Verification items for the finished model (mm, model axes). A direction names the side the tool comes from. Round coordinates to 2 decimals unless told otherwise and drop trailing zeros. Write each loop counter-clockwise with the first axis right and the second up, starting at its lowest first coordinate (ties: lowest second). Pieces come first, ordered by that corner, then holes. Notation, with made-up numbers: M 85,71 L 114,71 A29 ccw 114,97 Z; hole C 13,58 d6. An arc over 180 degrees is marked long. One line per item, written item: value. Start each with the question number.
Item 1: Section check B-B, the plane y = -67. Record the cut outline in (x, z), then the cut area to 3 significant figures.
Item 2: Thickness scan on probe 1 along Y at (x, z) = (13.5, -36); probe 2 along X at (y, z) = (-36, -20); probe 3 along Z at (x, y) = (26.5, -51.5). Record the ranges inside material, lowest first. Write a range as from..to.
Item 3: Gauge pin test, flat end, axial feed: pin 1 (8 mm diameter, centred on x = 18, y = -60.5, fed in from +Z). Record the tip position at first contact, or that the pin passes through.
Item 4: Section check C-C, the plane x = 21.5. Record the cut outline in (y, z).
Item 5: Tool access check on faces 1 (the face through (-10, -12.7, 1)), 2 (the face through (-13, -95, 48.157)). Record the directions out of +Z, -Z, +X, -X, +Y, -Y that give a thin tool (end or side, any length) a straight path to the whole face; none if there is none.
Item 6: Draft check along Y on faces 3 (the face through (-8.68, -1.45, 46.63)), 4 (the face through (-10, -50, -54.188)), 5 (the face through (30.67, -51.4, 46.71)), 6 (the face through (-10, -101.6, -2)). Enter one of: +Y half, -Y half, draft (parallel to the pull), parting line (faces both ways), or undercut.
Item 7: Section check A-A, the plane z = 18. Record the cut outline in (x, y).
from build123d import *

# Parameters (mm, degrees)
F0_W         = 102.3449450731
F0_H         = 102.3449450731
F1_DEPTH     = 101.6
F2_T         = -12.7
F3_R         = 5.08
F4_T1_DEPTH  = 92.1849450731
F4_T3_DEPTH  = 92.1849450731
F4_T5_DEPTH  = 91.44
F4_S9_W      = 5.08
F4_S9_H      = 5.08
F4_T10_DEPTH = 5.08
F4_S15_W     = 5.08
F4_S15_H     = 5.08
F4_T16_DEPTH = 5.08
F4_S21_W     = 5.08
F4_S21_H     = 5.08
F4_T22_DEPTH = 5.08
F4_S27_W     = 5.08
F4_S27_H     = 5.08
F4_T28_DEPTH = 5.08
F4_T32_ANGLE = 90
F4_T34_ANGLE = 90


# Not quite as in the source:
# - a fillet or chamfer that OpenCascade refuses, or shapes differently, is made with other operations: its cross-section is extruded or revolved along the edge and cut away or added


with BuildPart() as f1:
    # F0 (on Front) → F1 (new body)
    with BuildSketch(Plane.XZ):
        with Locations((-9.3297921121, -3.0156895518)):
            Rectangle(F0_W, F0_H)
    extrude(amount=F1_DEPTH)

    # F2
    f2_openings = [f1.faces().sort_by_distance(p)[0] for p in [
        (-9.329792, -50.8, 48.156783),
    ]]
    offset(amount=F2_T, openings=f2_openings)

    # F3
    f3_edges = [f1.edges().sort_by_distance(p)[0] for p in [
        (41.84268, -50.8, 48.156783),
        (-9.329792, -101.6, 48.156783),
        (41.84268, -101.6, -3.01569),
        (41.84268, -50.8, -54.188162),
        (-9.329792, -101.6, -54.188162),
        (-9.329792, -88.9, 48.156783),
        (-60.502265, -50.8, 48.156783),
        (-9.329792, 0, 48.156783),
        (29.14268, -50.8, 48.156783),
        (-9.329792, -12.7, 48.156783),
        (-47.802265, -50.8, 48.156783),
    ]]
    fillet(f3_edges, radius=F3_R)

    # F4: fillet of radius 5.08 on 3 edges, made by hand

    # F4_s2 → F4_t1 (cut)
    with BuildSketch(Plane.YZ.offset(-55.4222646487)):
        with BuildLine():
            ThreePointArc((-5.08, -54.1881620884), (-1.4878975516, -52.7002645368), (0, -49.1081620884))
            Line((0, -49.1081620884), (0, -54.1881620884))
            Line((0, -54.1881620884), (-5.08, -54.1881620884))
        make_face()
    extrude(amount=F4_T1_DEPTH, mode=Mode.SUBTRACT)

    # F4_s4 → F4_t3 (cut)
    with BuildSketch(Plane.XY.offset(-49.1081620884)):
        with BuildLine():
            ThreePointArc((-60.5022646487, -5.08), (-59.0143670971, -1.4878975516), (-55.4222646487, 0))
            Line((-55.4222646487, 0), (-60.5022646487, 0))
            Line((-60.5022646487, 0), (-60.5022646487, -5.08))
        make_face()
        with BuildLine():
            ThreePointArc((-60.5022646487, -96.52), (-59.0143670971, -100.1121024484), (-55.4222646487, -101.6))
            Line((-55.4222646487, -101.6), (-60.5022646487, -101.6))
            Line((-60.5022646487, -101.6), (-60.5022646487, -96.52))
        make_face()
        with BuildLine():
            ThreePointArc((36.7626804245, 0), (40.3547828729, -1.4878975516), (41.8426804245, -5.08))
            Line((41.8426804245, -5.08), (41.8426804245, 0))
            Line((41.8426804245, 0), (36.7626804245, 0))
        make_face()
    extrude(amount=F4_T3_DEPTH, mode=Mode.SUBTRACT)

    # F4_s6 → F4_t5 (cut)
    with BuildSketch(Plane.XZ.offset(5.08)):
        with BuildLine():
            ThreePointArc((-60.5022646487, -49.1081620884), (-59.0143670971, -52.7002645368), (-55.4222646487, -54.1881620884))
            Line((-55.4222646487, -54.1881620884), (-60.5022646487, -54.1881620884))
            Line((-60.5022646487, -54.1881620884), (-60.5022646487, -49.1081620884))
        make_face()
    extrude(amount=F4_T5_DEPTH, mode=Mode.SUBTRACT)


with BuildPart() as f4_tool8:
    # F4_s9 → F4_t10 (new body)
    with BuildSketch(Plane.YZ.offset(-55.4222646487)):
        with Locations((-99.06, 45.6167829847)):
            Rectangle(F4_S9_W, F4_S9_H)
    extrude(amount=-F4_T10_DEPTH)

    # F4_s11 → F4_t12 (revolve, cut)
    with BuildSketch(Plane(origin=(-55.4222646487, -96.52, 43.0767829847), x_dir=(0, 0.7071067812, -0.7071067812), z_dir=(0, 0.7071067812, 0.7071067812))):
        with BuildLine():
            ThreePointArc((0, -5.08), (5.08, 0), (0, 5.08))
            Line((0, 5.08), (0, -5.08))
        make_face()
    revolve(axis=Axis((-55.4222646487, -96.52, 43.0767829847), (-1, 0, 0)), mode=Mode.SUBTRACT)


with BuildPart() as f1_1:
    add(f1.part)

    # F4_t7: cut F4_tool8
    add(f4_tool8.part, mode=Mode.SUBTRACT)


with BuildPart() as f4_tool14:
    # F4_s15 → F4_t16 (new body)
    with BuildSketch(Plane.YZ.offset(-55.4222646487)):
        with Locations((-2.54, 45.6167829847)):
            Rectangle(F4_S15_W, F4_S15_H)
    extrude(amount=-F4_T16_DEPTH)

    # F4_s17 → F4_t18 (revolve, cut)
    with BuildSketch(Plane(origin=(-55.4222646487, -5.08, 43.0767829847), x_dir=(0, -0.7071067812, -0.7071067812), z_dir=(0, 0.7071067812, -0.7071067812))):
        with BuildLine():
            ThreePointArc((0, -5.08), (5.08, 0), (0, 5.08))
            Line((0, 5.08), (0, -5.08))
        make_face()
    revolve(axis=Axis((-55.4222646487, -5.08, 43.0767829847), (-1, 0, 0)), mode=Mode.SUBTRACT)


with BuildPart() as f1_2:
    add(f1_1.part)

    # F4_t13: cut F4_tool14
    add(f4_tool14.part, mode=Mode.SUBTRACT)


with BuildPart() as f4_tool20:
    # F4_s21 → F4_t22 (new body)
    with BuildSketch(Plane.XZ.offset(5.08)):
        with Locations((39.3026804245, 45.6167829847)):
            Rectangle(F4_S21_W, F4_S21_H)
    extrude(amount=-F4_T22_DEPTH)

    # F4_s23 → F4_t24 (revolve, cut)
    with BuildSketch(Plane(origin=(36.7626804245, -5.08, 43.0767829847), x_dir=(-0.7071067812, 0, -0.7071067812), z_dir=(0.7071067812, 0, -0.7071067812))):
        with BuildLine():
            ThreePointArc((0, -5.08), (5.08, 0), (0, 5.08))
            Line((0, 5.08), (0, -5.08))
        make_face()
    revolve(axis=Axis((36.7626804245, -5.08, 43.0767829847), (0, 1, 0)), mode=Mode.SUBTRACT)


with BuildPart() as f1_3:
    add(f1_2.part)

    # F4_t19: cut F4_tool20
    add(f4_tool20.part, mode=Mode.SUBTRACT)


with BuildPart() as f4_tool26:
    # F4_s27 → F4_t28 (new body)
    with BuildSketch(Plane.YZ.offset(-55.4222646487)):
        with Locations((-2.54, -51.6481620884)):
            Rectangle(F4_S27_W, F4_S27_H)
    extrude(amount=-F4_T28_DEPTH)

    # F4_s29 → F4_t30 (revolve, cut)
    with BuildSketch(Plane(origin=(-55.4222646487, -5.08, -49.1081620884), x_dir=(0, -0.7071067812, 0.7071067812), z_dir=(0, -0.7071067812, -0.7071067812))):
        with BuildLine():
            ThreePointArc((0, -5.08), (5.08, 0), (0, 5.08))
            Line((0, 5.08), (0, -5.08))
        make_face()
    revolve(axis=Axis((-55.4222646487, -5.08, -49.1081620884), (-1, 0, 0)), mode=Mode.SUBTRACT)


with BuildPart() as f1_4:
    add(f1_3.part)

    # F4_t25: cut F4_tool26
    add(f4_tool26.part, mode=Mode.SUBTRACT)

    # F4_s31 → F4_t32 (revolve, cut)
    with BuildSketch(Plane.XZ.offset(96.52)):
        with BuildLine():
            ThreePointArc((-60.5022646487, -49.1081620884), (-59.0143670971, -52.7002645368), (-55.4222646487, -54.1881620884))
            Line((-55.4222646487, -54.1881620884), (-60.5022646487, -54.1881620884))
            Line((-60.5022646487, -54.1881620884), (-60.5022646487, -49.1081620884))
        make_face()
    revolve(axis=Axis((-60.5022646487, -96.52, -49.1081620884), (-1, 0, 0)), revolution_arc=F4_T32_ANGLE, mode=Mode.SUBTRACT)

    # F4_s33 → F4_t34 (revolve, cut)
    with BuildSketch(Plane.YZ.offset(36.7626804245)):
        with BuildLine():
            ThreePointArc((0, -49.1081620884), (-1.4878975516, -52.7002645368), (-5.08, -54.1881620884))
            Line((-5.08, -54.1881620884), (0, -54.1881620884))
            Line((0, -54.1881620884), (0, -49.1081620884))
        make_face()
    revolve(axis=Axis((36.7626804245, 0, -49.1081620884), (0, -1, 0)), revolution_arc=F4_T34_ANGLE, mode=Mode.SUBTRACT)


solid = f1_4.part
Response values:
1. outline: M -60.5,-49.11 A5.08 ccw -55.42,-54.19 L 36.76,-54.19 A5.08 ccw 41.84,-49.11 L 41.84,43.08 A5.08 ccw 36.76,48.16 L 34.22,48.16 A5.08 ccw 29.14,43.08 L 29.14,-41.49 L -47.8,-41.49 L -47.8,43.08 A5.08 ccw -52.88,48.16 L -55.42,48.16 A5.08 ccw -60.5,43.08 Z
1. area: 3,540 mm2
2. probe 1: y = -101.6..-88.9, -12.7..0
2. probe 2: x = -60.5..-47.8, 29.14..41.84
2. probe 3: z = -54.19..-41.49
3. pin 1: stops at z = -41.49
4. outline: M -101.6,-49.11 A5.08 ccw -96.52,-54.19 L -5.08,-54.19 A5.08 ccw 0,-49.11 L 0,43.08 A5.08 ccw -5.08,48.16 L -7.62,48.16 A5.08 ccw -12.7,43.08 L -12.7,-41.49 L -88.9,-41.49 L -88.9,43.08 A5.08 ccw -93.98,48.16 L -96.52,48.16 A5.08 ccw -101.6,43.08 Z
5. face 1: +Z
5. face 2: +Z, +X, -X, +Y, -Y
6. face 3: +Y half
6. face 4: draft
6. face 5: undercut
6. face 6: -Y half
7. outline: M -60.5,-96.52 A5.08 ccw -55.42,-101.6 L 36.76,-101.6 A5.08 ccw 41.84,-96.52 L 41.84,-5.08 A5.08 ccw 36.76,0 L -55.42,0 A5.08 ccw -60.5,-5.08 Z; hole M -47.8,-88.9 L 29.14,-88.9 L 29.14,-12.7 L -47.8,-12.7 Z
